```python
from build123d import *

# Parameters (mm, degrees)
SKETCH1_W           = 187.5
SKETCH1_H           = 20
BOSS_EXTRUDE1_DEPTH = 100
SKETCH2_W           = 8.1
SKETCH2_H           = 5.3
CUT_EXTRUDE1_DEPTH  = 100
SKETCH3_R           = 1.75
CUT_EXTRUDE2_DEPTH  = 8
CHAMFER1_SIZE       = 0.5
CHAMFER2_SIZE       = 0.5
SKETCH4_W           = 15
SKETCH4_H           = 2
BOSS_EXTRUDE2_DEPTH = 15
SKETCH5_W           = 15
SKETCH5_H           = 2
BOSS_EXTRUDE3_DEPTH = 15
SKETCH6_R           = 2.15
CUT_EXTRUDE3_DEPTH  = 15
CHAMFER3_SIZE       = 1


with BuildPart() as part:
    # Sketch1 → Boss-Extrude1 (new body)
    with BuildSketch(Plane(origin=(0, 0, 0), x_dir=(1, 0, 0), z_dir=(0, 1, 0))):
        with Locations((93.75, 10)):
            Rectangle(SKETCH1_W, SKETCH1_H)
    extrude(amount=BOSS_EXTRUDE1_DEPTH)

    # Sketch2 → Cut-Extrude1 (cut)
    with BuildSketch(Plane(origin=(0, 100, 0), x_dir=(1, 0, 0), z_dir=(0, 1, 0))):
        with Locations((4.05, 10)):
            Rectangle(SKETCH2_W, SKETCH2_H)
        with Locations((183.45, 10)):
            Rectangle(SKETCH2_W, SKETCH2_H)
    extrude(amount=-CUT_EXTRUDE1_DEPTH, mode=Mode.SUBTRACT)

    # Sketch3 → Cut-Extrude2 (cut)
    with BuildSketch(Plane(origin=(0, 100, 0), x_dir=(1, 0, 0), z_dir=(0, 1, 0))):
        with Locations(Location((40.1, 10, 0), (0, 0, 270))):
            Circle(SKETCH3_R)
        with Locations(Location((135, 10, 0), (0, 0, 270))):
            Circle(SKETCH3_R)
    extrude(amount=-CUT_EXTRUDE2_DEPTH, mode=Mode.SUBTRACT)

    # Chamfer1
    chamfer1_edges = [part.edges().sort_by_distance(p)[0] for p in [
        (40.1, 100, -11.75),
    ]]
    chamfer(chamfer1_edges, length=CHAMFER1_SIZE)

    # Chamfer2
    chamfer2_edges = [part.edges().sort_by_distance(p)[0] for p in [
        (135, 100, -11.75),
    ]]
    chamfer(chamfer2_edges, length=CHAMFER2_SIZE)

    # Sketch4 → Boss-Extrude2 (add)
    with BuildSketch(Plane(origin=(0, 0, -20), x_dir=(-1, 0, 0), z_dir=(0, 0, -1))):
        with Locations((-93.75, 1)):
            Rectangle(SKETCH4_W, SKETCH4_H)
    extrude(amount=BOSS_EXTRUDE2_DEPTH)

    # Sketch5 → Boss-Extrude3 (add)
    with BuildSketch(Plane.XY):
        with Locations((93.75, 1)):
            Rectangle(SKETCH5_W, SKETCH5_H)
    extrude(amount=BOSS_EXTRUDE3_DEPTH)

    # Sketch6 → Cut-Extrude3 (cut)
    with BuildSketch(Plane(origin=(0, 2, 0), x_dir=(1, 0, 0), z_dir=(0, 1, 0))):
        with Locations(Location((93.75, 27.5, 0), (0, 0, 180))):
            Circle(SKETCH6_R)
        with Locations(Location((93.75, -7.5, 0), (0, 0, 180))):
            Circle(SKETCH6_R)
    extrude(amount=-CUT_EXTRUDE3_DEPTH, mode=Mode.SUBTRACT)

    # Chamfer3
    chamfer3_edges = [part.edges().sort_by_distance(p)[0] for p in [
        (95.9, 2, -27.5),
        (95.9, 2, 7.5),
    ]]
    chamfer(chamfer3_edges, length=CHAMFER3_SIZE)


solid = part.part
```
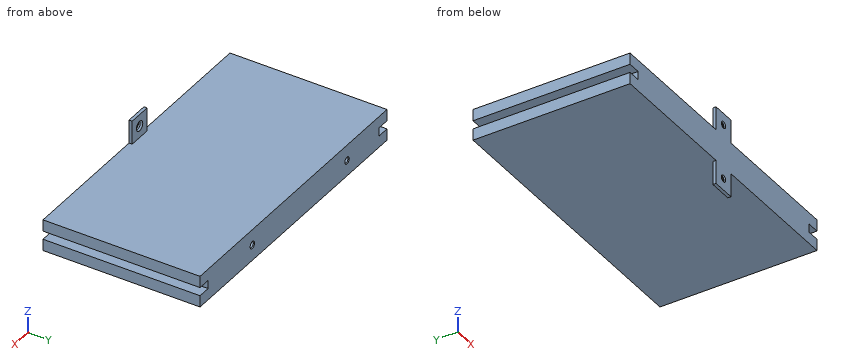
Here's how the part is built. I have some questions about the finished solid (model axes, mm). Coordinates: 2 decimals unless noted, no trailing zeros. Order: outer loops, then holes, each group sorted by start corner. A loop starts at its lowest first (then second) coordinate and runs counter-clockwise, first axis right, second up.
1) Will these pins go through, and if not, where does the flat tip stop? pin 1 (5 mm diameter, centred on x = 117, y = 37.5, fed in from -Z); pin 2 (1.6 mm diameter, centred on y = 1.5, z = -28, fed in from +X); pin 3 (3 mm diameter, centred on x = 135, z = -10, fed in from -Y); pin 4 (3 mm diameter, centred on x = 40.1, z = -10, fed in from +Y).
2) I need wall thicknesses on line 1 (Z direction, x = 93.75, y = 0.2); line 2 (X direction, y = 97.5, z = -10); line 3 (Z direction, x = 135, y = 95.5). Which ranges of each line are inside material? Lowest first, please.
3) Imagine slicing it at B-B on x = 93.75. List the corners of the cut face in (y, z) for me, and give its area (3 significant figures).
4) Imagine slicing it at C-C on y = 66.5. List the corners of the cut face in (x, z) for me.
5) Imagine slicing it at A-A on z = -27.5. List the corners of the cut face in (x, y) for me.
6) Imagine slicing it at D-D on z = -10. List the corners of the cut face in (x, y) for me, and give its area (3 significant figures).
Response values:
1. pin 1: stops at z = -20
1. pin 2: stops at x = 101.25
1. pin 3: stops at y = 0
1. pin 4: stops at y = 92
2. line 1: z = -35 to -29.65, -25.35 to 5.35, 9.65 to 15
2. line 2: x = 8.1 to 38.35, 41.85 to 133.25, 136.75 to 179.4
2. line 3: z = -20 to -11.75, -8.25 to 0
3. outline: (0, -35) - (2, -35) - (2, -30.65) - (1, -29.65) - (0, -29.65) - close; (0, -25.35) - (1, -25.35) - (2, -24.35) - (2, -20) - (100, -20) - (100, 0) - (2, 0) - (2, 4.35) - (1, 5.35) - (0, 5.35) - close; (0, 9.65) - (1, 9.65) - (2, 10.65) - (2, 15) - (0, 15) - close
3. area: 2,040 mm2
4. outline: (0, -20) - (187.5, -20) - (187.5, -12.65) - (179.4, -12.65) - (179.4, -7.35) - (187.5, -7.35) - (187.5, 0) - (0, 0) - (0, -7.35) - (8.1, -7.35) - (8.1, -12.65) - (0, -12.65) - close
5. outline: (86.25, 0) - (91.6, 0) - (91.6, 1) - (90.6, 2) - (86.25, 2) - close; (95.9, 0) - (101.25, 0) - (101.25, 2) - (96.9, 2) - (95.9, 1) - close
6. outline: (8.1, 0) - (179.4, 0) - (179.4, 100) - (137.25, 100) - (136.75, 99.5) - (136.75, 92) - (133.25, 92) - (133.25, 99.5) - (132.75, 100) - (42.35, 100) - (41.85, 99.5) - (41.85, 92) - (38.35, 92) - (38.35, 99.5) - (37.85, 100) - (8.1, 100) - close
6. area: 17,100 mm2
